Job drawing, mm, ordinate dimensions from the low corner. One solid piece. Round coordinates to 2 decimals unless told otherwise and drop trailing zeros. Loops run counter-clockwise (first coordinate to the right, second up) from the corner with the lowest first, then second, coordinate; pieces in that order, holes last. Notation, with made-up numbers: M 40.5,30.25 L 57.5,30.25 A20 ccw 57.5,39.25 Z; hole C 66.25,-24 d4. An arc over 180 degrees is marked long. One line per item, written item: value.
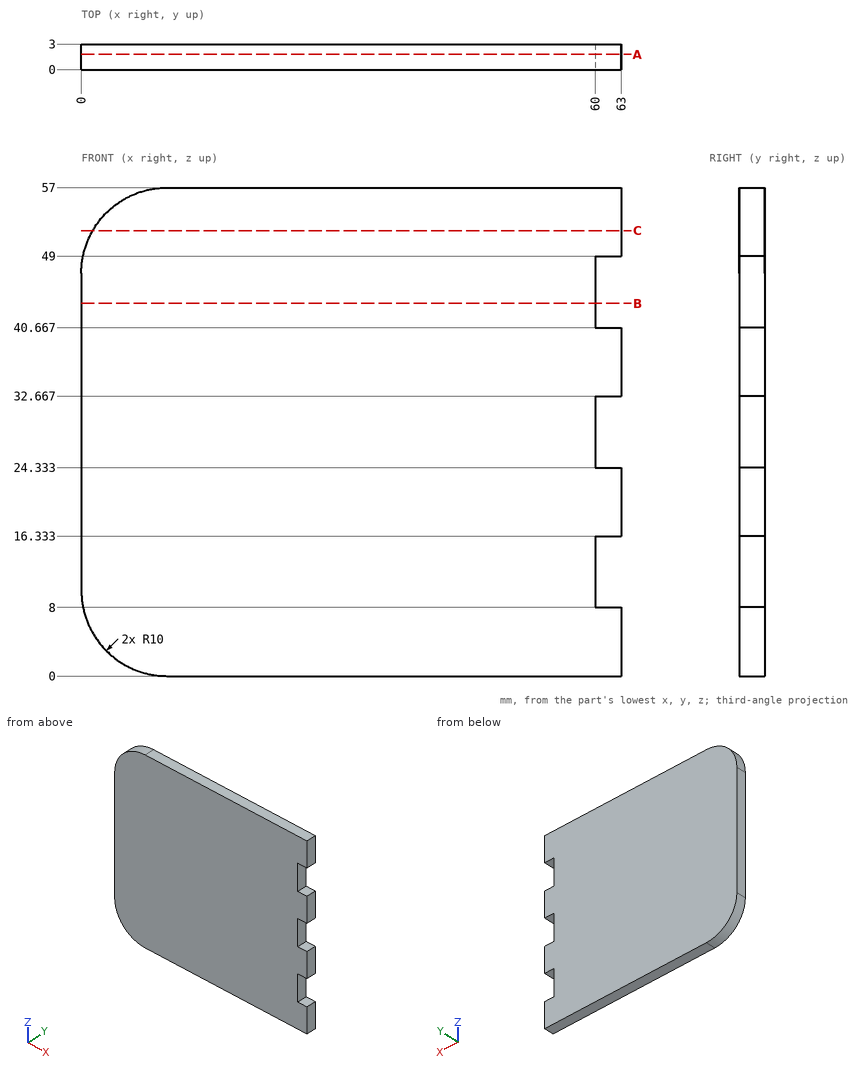
Item 1: Wall check: line 1 along X through (y, z) = (2.85, 14.5); line 2 along X through (y, z) = (0.9, 48); line 3 along Z through (x, y) = (6, 0.4) (1 decimal). Give the ranges that are in metal, low to high.
Check values:
line 1: x = 0 to 60
line 2: x = 0.05 to 60
line 3: z = 0.8 to 56.2
Item 2: Slice it at A-A, the plane y = 1.8. Give the cut face in (x, z).
Check values:
outline: M 0,10 A10 ccw 10,0 L 63,0 L 63,8 L 60,8 L 60,16.33 L 63,16.33 L 63,24.33 L 60,24.33 L 60,32.67 L 63,32.67 L 63,40.67 L 60,40.67 L 60,49 L 63,49 L 63,57 L 10,57 A10 ccw 0,47 Z
Item 3: Slice it at B-B, the plane z = 43.5. Give the cut face in (x, y), and give its area (3 significant figures).
Check values:
outline: M 0,0 L 60,0 L 60,3 L 0,3 Z
area: 180 mm2
Item 4: Slice it at C-C, the plane z = 52. Give the cut face in (x, y).
Check values:
outline: M 1.34,0 L 63,0 L 63,3 L 1.34,3 Z
Item 5: Drop a flat-ended pin along its axis: P1, Ø0.9, axis at y = 1.5, z = 13, coming from the +X side. Give the stop position or say it passes through.
Check values:
P1: stops at x = 60
